```python
from build123d import *

# Parameters (mm, degrees)
ESTRUSIONE_ESTRUSIONE1_DEPTH = 5
SCHIZZO2_R                   = 1.5
SCHIZZO2_R_2                 = 2
TAGLIO_ESTRUSIONE1_DEPTH     = 6


with BuildPart() as part:
    # Schizzo1 → Estrusione-Estrusione1 (new body)
    with BuildSketch(Plane(origin=(0, 0, 0), x_dir=(0, 0, -1), z_dir=(1, 0, 0))):
        with BuildLine():
            Line((-5, 10), (5, 10))
            ThreePointArc((5, 10), (15, 0), (5, -10))
            Line((5, -10), (-5, -10))
            ThreePointArc((-5, -10), (-15, 0), (-5, 10))
        make_face()
    extrude(amount=ESTRUSIONE_ESTRUSIONE1_DEPTH)

    # Schizzo2 → Taglio-Estrusione1 (cut, through all)
    with BuildSketch(Plane(origin=(0, 0, 0), x_dir=(0, 0, -1), z_dir=(1, 0, 0))):
        with Locations((-5, 7)):
            Circle(SCHIZZO2_R)
        Circle(SCHIZZO2_R_2)
        with Locations((5, 7)):
            Circle(SCHIZZO2_R)
        with Locations((-5, -7)):
            Circle(SCHIZZO2_R)
        with Locations((5, -7)):
            Circle(SCHIZZO2_R)
    extrude(amount=TAGLIO_ESTRUSIONE1_DEPTH, mode=Mode.SUBTRACT)


solid = part.part
```
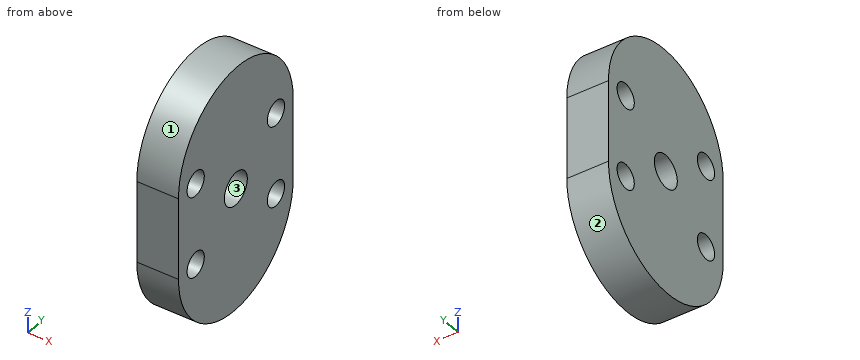
Geometry check sheet. Reference: the model listing, model coordinates, mm. Face numbers are marked on the shaded views. Coordinates: 2 decimals unless noted, no trailing zeros. Order: outer loops, then holes, each group sorted by start corner. A loop starts at its lowest first (then second) coordinate and runs counter-clockwise, first axis right, second up. Notation, with made-up numbers: M 28,75 L 53,75 A19 cw 53,85 Z; hole C 81.25,-30 d10. An arc over 180 degrees is marked long. Answer as a JSON object with one key per item and string values.
Q1. Cross-section at D-D on y = -7. Record the cut outline in (x, z), and give its area (3 significant figures).
Results are:
{"outline": "M 0,-12.14 L 5,-12.14 L 5,-6.5 L 0,-6.5 Z; M 0,-3.5 L 5,-3.5 L 5,3.5 L 0,3.5 Z; M 0,6.5 L 5,6.5 L 5,12.14 L 0,12.14 Z", "area": "91.4 mm²"}
Q2. Scan lines: line 1 (Y direction, x = 1.05, z = 5); line 2 (Z direction, x = 4.05, y = 7); line 3 (Z direction, x = 1.55, y = -6.25). Record each from-to range of solid material in increasing order.
Results are:
{"line 1": "y = -10 to -8.5, -5.5 to 5.5, 8.5 to 10", "line 2": "z = -12.14 to -6.5, -3.5 to 3.5, 6.5 to 12.14", "line 3": "z = -12.81 to -6.3, -3.7 to 3.7, 6.3 to 12.81"}
Q3. Cross-section at B-B on z = 0. Record the cut outline in (x, y).
Results are:
{"outline": "M 0,-10 L 5,-10 L 5,-2 L 0,-2 Z; M 0,2 L 5,2 L 5,10 L 0,10 Z"}
Q4. Cross-section at A-A on y = 0. Record the cut outline in (x, z), and give its area (3 significant figures).
Results are:
{"outline": "M 0,-15 L 5,-15 L 5,-2 L 0,-2 Z; M 0,2 L 5,2 L 5,15 L 0,15 Z", "area": "130 mm²"}
Q5. Release check for a two-part mould opening along Z. For the marked faces 1, 2 and 3 record: released by +Z, released by -Z, zero draft, split by the parting line, or undercut.
Results are:
{"face 1": "released by +Z", "face 2": "released by -Z", "face 3": "undercut"}
Q6. Depth check by flat-ended pin: pin 1 Ø2 at (x, y) = (2, -6.5) entering from +Z. Enter the tip coordinate at first touch or a pass-through.
Results are:
{"pin 1": "stops at z = 13.35"}
Q7. Cross-section at C-C on x = 3.7. Record the cut outline in (y, z).
Results are:
{"outline": "M -10,-5 A10 ccw 10,-5 L 10,5 A10 ccw -10,5 Z; hole C -7,-5 d3; hole C -7,5 d3; hole C 0,0 d4; hole C 7,-5 d3; hole C 7,5 d3"}
